Design review of the part built by this model. Coordinates are the model's own, in mm. A direction names the side the tool comes from. Give positions to 0.01 mm unless a question says otherwise; leave off trailing zeros. Write each loop counter-clockwise with the first axis right and the second up, starting at its lowest first coordinate (ties: lowest second). Pieces come first, ordered by that corner, then holes. Notation, with made-up numbers: (-5, 24) -> (11, 24) arc R25 cw to (11, 46) -> close; hole circle Ø5 at (-31, -18.75). An arc over 180 degrees is marked (long way). Write each question's results on one line, items separated by ' | '. Start each with the question number.
(1) Mouldability with a two-part tool opening along X and no side actions: class faces 4 (the face through (113, 0, 0)), 5 (the face through (77.65, 0.53, 11.99)), 6 (the face through (20, 8.2, 0)) as released by +X, released by -X, zero draft, split by the parting line, or undercut.
(2) Clearance check with flat-ended pins moving along their axes: pin 1 (2 mm diameter, centred on x = 55.5, z = -10.5, fed in from -Y); pin 2 (6 mm diameter, centred on x = 77, y = -7.5, fed in from -Z); pin 3 (4 mm diameter, centred on x = 99.5, z = 5, fed in from +Y). State where each tip first meets the part, or that it passes through.
(3) To check wall thickness, follow probe 1 along X at (y, z) = (11, -1.5); probe 2 along X at (y, z) = (1, 11.5); probe 3 along X at (y, z) = (14, -2.5). State the ranges of each line that lie inside material, in increasing order.
(4) Take a section at A-A (y = 7). State the section outline as (x, z) points.
(5) For faces 1 (the face through (53, 4, -11)), 2 (the face through (88, -2, 6)), 3 (the face through (102.65, -7.81, 1.73)), list the 3-axis set-ups (+Z, -Z, +X, -X, +Y, -Y) from which the entire face can be reached by the end or side of a thin tool; tool diameter is ignored.
(6) Take a section at C-C (x = 69). State the section outline as (y, z) points, plus the area to 3 significant figures.
from build123d import *

# Parameters (mm, degrees)
F0_W   = 4
F0_H   = 8
F0_H_2 = 10
F0_H_3 = 6


with BuildPart() as f1:
    # F0 (on Front) → F1 (revolve)
    with BuildSketch(Plane.XZ):
        Polygon((20, 0), (0, 0), (0, -10), (20, -10), (20, -8), align=None)
        with Locations((22, -4)):
            Rectangle(F0_W, F0_H)
        Polygon((53, 0), (24, 0), (24, -8), (24, -11.5), (53, -11.5), align=None)
        Polygon((63, 0), (53, 0), (53, -11.5), (53, -16), (63, -16), (63, -10), align=None)
        with Locations((65, -5)):
            Rectangle(F0_W, F0_H_2)
        Polygon((88, 0), (67, 0), (67, -10), (67, -12), (88, -12), (88, -6), align=None)
        with Locations((90, -3)):
            Rectangle(F0_W, F0_H_3)
        Polygon((113, 0), (92, 0), (92, -6), (92, -8), (113, -8), align=None)
    revolve(axis=Axis((38.5, 0, 0), (1, 0, 0)))


solid = f1.part
Report:
1) face 4: released by +X | face 5: zero draft | face 6: undercut
2) pin 1: y = -12.87 | pin 2: z = -11.12 | pin 3: y = 7.42
3) probe 1: 24 to 63, 67 to 88 | probe 2: 53 to 63, 67 to 88 | probe 3: 53 to 63
4) outline: (0, -7.14) -> (20, -7.14) -> (20, -3.87) -> (24, -3.87) -> (24, -9.12) -> (53, -9.12) -> (53, -14.39) -> (63, -14.39) -> (63, -7.14) -> (67, -7.14) -> (67, -9.75) -> (88, -9.75) -> (88, 9.75) -> (67, 9.75) -> (67, 7.14) -> (63, 7.14) -> (63, 14.39) -> (53, 14.39) -> (53, 9.12) -> (24, 9.12) -> (24, 3.87) -> (20, 3.87) -> (20, 7.14) -> (0, 7.14) -> close; (92, -3.87) -> (113, -3.87) -> (113, 3.87) -> (92, 3.87) -> close
5) face 1: -X | face 2: none | face 3: +X
6) outline: circle Ø24 at (0, 0) | area: 452 mm2
